Verification items for the finished model (mm, model axes). A direction names the side the tool comes from. Give positions to 0.01 mm unless a question says otherwise; leave off trailing zeros. Write each loop counter-clockwise with the first axis right and the second up, starting at its lowest first coordinate (ties: lowest second). Pieces come first, ordered by that corner, then holes.
from build123d import *

# Parameters (mm, degrees)
SKETCH1_W           = 36
SKETCH1_H           = 28.5
SKETCH1_R           = 1.7
SKETCH1_R_2         = 5
SKETCH1_W_2         = 9
BOSS_EXTRUDE2_DEPTH = 3
SKETCH2_W           = 4
SKETCH2_H           = 20.5
BOSS_EXTRUDE3_DEPTH = 21.75
SKETCH4_R           = 10.25
BOSS_EXTRUDE4_DEPTH = 4
SKETCH6_R           = 4.4
SKETCH6_R_2         = 1.2
CUT_EXTRUDE3_DEPTH  = 4


with BuildPart() as part:
    # Sketch1 → Boss-Extrude2 (new body)
    # profile 1 of 3: a face of its own
    with BuildSketch(Plane(origin=(0, 0, 0), x_dir=(1, 0, 0), z_dir=(0, 1, 0))):
        Rectangle(SKETCH1_W, SKETCH1_H)
        with Locations(Location((-9, -8.25, 0), (0, 0, 270))):
            Circle(SKETCH1_R, mode=Mode.SUBTRACT)
        with Locations(Location((9, -8.25, 0), (0, 0, 270))):
            Circle(SKETCH1_R, mode=Mode.SUBTRACT)
        with Locations(Location((-9, 8.25, 0), (0, 0, 270))):
            Circle(SKETCH1_R, mode=Mode.SUBTRACT)
        with Locations(Location((0, 0, 0), (0, 0, 270))):
            Circle(SKETCH1_R_2, mode=Mode.SUBTRACT)
        with Locations(Location((9, 8.25, 0), (0, 0, 270))):
            Circle(SKETCH1_R, mode=Mode.SUBTRACT)
    # profile 2 of 3: a face of its own
    with BuildSketch(Plane(origin=(0, 0, 0), x_dir=(1, 0, 0), z_dir=(0, 1, 0))):
        with Locations((-22.5, 0)):
            Rectangle(SKETCH1_W_2, SKETCH1_H)
    # profile 3 of 3: a face of its own
    with BuildSketch(Plane(origin=(0, 0, 0), x_dir=(1, 0, 0), z_dir=(0, 1, 0))):
        with Locations((22.5, 0)):
            Rectangle(SKETCH1_W_2, SKETCH1_H)
    extrude(amount=BOSS_EXTRUDE2_DEPTH)

    # Sketch2 → Boss-Extrude3 (add)
    with BuildSketch(Plane(origin=(0, 3, 0), x_dir=(1, 0, 0), z_dir=(0, 1, 0))):
        with Locations((25, 0)):
            Rectangle(SKETCH2_W, SKETCH2_H)
    boss_extrude3 = extrude(amount=BOSS_EXTRUDE3_DEPTH)

    # Sketch4 → Boss-Extrude4 (add)
    with BuildSketch(Plane(origin=(27, 0, 0), x_dir=(0, 0, -1), z_dir=(1, 0, 0))):
        with Locations((0, 24.75)):
            Circle(SKETCH4_R)
    boss_extrude4 = extrude(amount=-BOSS_EXTRUDE4_DEPTH)

    # Mirror1: Boss-Extrude3, Boss-Extrude4 across plane
    add(boss_extrude3.mirror(Plane(origin=(0, 0, 0), x_dir=(0, 0, 1), z_dir=(1, 0, 0))))
    add(boss_extrude4.mirror(Plane(origin=(0, 0, 0), x_dir=(0, 0, 1), z_dir=(1, 0, 0))))

    # Sketch6 → Cut-Extrude3 (cut)
    with BuildSketch(Plane(origin=(27, 0, 0), x_dir=(0, 0, -1), z_dir=(1, 0, 0))):
        with Locations((0, 24.75)):
            Circle(SKETCH6_R)
        with Locations((0, 32.75)):
            Circle(SKETCH6_R_2)
        with Locations((8, 24.75)):
            Circle(SKETCH6_R_2)
        with Locations((0, 16.75)):
            Circle(SKETCH6_R_2)
        with Locations((-8, 24.75)):
            Circle(SKETCH6_R_2)
    cut_extrude3 = extrude(amount=-CUT_EXTRUDE3_DEPTH, mode=Mode.SUBTRACT)

    # Mirror3: Cut-Extrude3 across plane
    add(cut_extrude3.mirror(Plane(origin=(0, 0, 0), x_dir=(0, 0, 1), z_dir=(1, 0, 0))), mode=Mode.SUBTRACT)


solid = part.part
Item 1: Scan lines: line 1 along X through (y, z) = (1.4, -8.25); line 2 along Y through (x, z) = (-23.9, 0); line 3 along X through (y, z) = (33, 2). Record each from-to range of solid material in increasing order.
Answer key:
line 1: x = -27 to -10.7, -7.3 to 7.3, 10.7 to 27
line 2: y = 0 to 15.55, 17.95 to 20.35, 29.15 to 31.55, 33.95 to 35
line 3: x = -27 to -23, 23 to 27
Item 2: Sectioned sample at C-C on z = -8. Record the cut outline in (x, y), then the cut area to 3 significant figures.
Answer key:
outline: (-27, 0) - (-10.68, 0) - (-10.68, 3) - (-23, 3) - (-23, 23.55) - (-27, 23.55) - close; (-27, 25.95) - (-23, 25.95) - (-23, 31.16) - (-27, 31.16) - close; (-7.32, 0) - (7.32, 0) - (7.32, 3) - (-7.32, 3) - close; (10.68, 0) - (27, 0) - (27, 23.55) - (23, 23.55) - (23, 3) - (10.68, 3) - close; (23, 25.95) - (27, 25.95) - (27, 31.16) - (23, 31.16) - close
area: 348 mm2
Item 3: Sectioned sample at A-A on x = -9. Record the cut outline in (y, z), then the cut area to 3 significant figures.
Answer key:
outline: (0, -14.25) - (3, -14.25) - (3, -9.95) - (0, -9.95) - close; (0, -6.55) - (3, -6.55) - (3, 6.55) - (0, 6.55) - close; (0, 9.95) - (3, 9.95) - (3, 14.25) - (0, 14.25) - close
area: 65.1 mm2
Item 4: Depth check by flat-ended pin: pin 1 (5.5 mm diameter, centred on x = -9, z = -8.25, fed in from +Y); pin 2 (2 mm diameter, centred on x = -25, y = 16.5, fed in from -Z); pin 3 (1.9 mm diameter, centred on y = 32.75, z = 0, fed in from +X); pin 4 (1.2 mm diameter, centred on x = -24.5, y = 10.5, fed in from +Z). Enter the tip coordinate at first touch or a pass-through.
Answer key:
pin 1: stops at y = 3
pin 2: stops at z = -10.25
pin 3: passes through
pin 4: stops at z = 10.25
Item 5: Sectioned sample at B-B on y = 16.75. Record the cut outline in (x, z), then the cut area to 3 significant figures.
Answer key:
outline: (-27, -10.25) - (-23, -10.25) - (-23, -1.2) - (-27, -1.2) - close; (-27, 1.2) - (-23, 1.2) - (-23, 10.25) - (-27, 10.25) - close; (23, -10.25) - (27, -10.25) - (27, -1.2) - (23, -1.2) - close; (23, 1.2) - (27, 1.2) - (27, 10.25) - (23, 10.25) - close
area: 145 mm2
Item 6: Sectioned sample at D-D on z = 0. State how many separate pieces and enclosed holes the cut face has, then the cut area to 3 significant figures.
Answer key:
separate pieces: 8
enclosed holes: 0
area: 279 mm2
Item 7: Release check for a two-part mould opening along Z. For faces 4 (the face through (0, 1, -14.25)), 5 (the face through (-6, 0, 0)), 6 (the face through (-25.03, 15.58, 0.26)), 7 (the face through (25.03, 15.58, 0.26)) record: released by +Z, released by -Z, zero draft, split by the parting line, or undercut.
Answer key:
face 4: released by -Z
face 5: zero draft
face 6: undercut
face 7: undercut
Item 8: Set-up check for faces 1 (the face through (25, 14, -10.25)), 2 (the face through (-25, 14, 10.25)), 3 (the face through (23, 19, 0)): record each of +Z, -Z, +X, -X, +Y, -Y from which the full face is reachable in a straight line by a thin tool's end or side.
Answer key:
face 1: -Z, +X, -X, +Y
face 2: +Z, +X, -X, +Y
face 3: +Z, -Z, +Y
